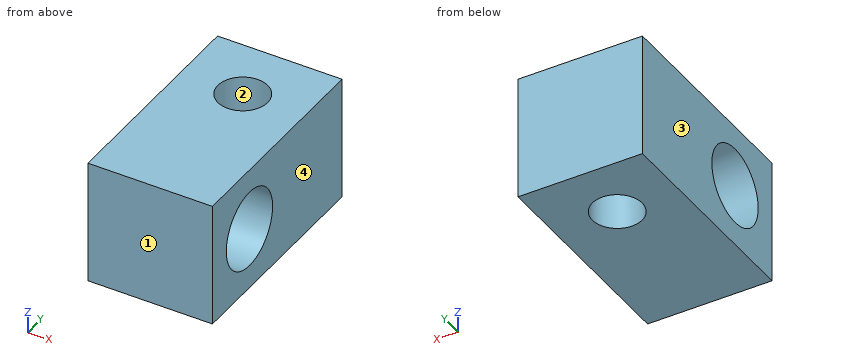
from build123d import *

# Parameters (mm, degrees)
SKETCH1_W           = 8
SKETCH1_H           = 14
BOSS_EXTRUDE1_DEPTH = 8
SKETCH2_R           = 1.6
CUT_EXTRUDE1_DEPTH  = 9
SKETCH4_R           = 2.5
CUT_EXTRUDE2_DEPTH  = 9


with BuildPart() as part:
    # Sketch1 → Boss-Extrude1 (new body)
    with BuildSketch(Plane.XY):
        Rectangle(SKETCH1_W, SKETCH1_H)
    extrude(amount=BOSS_EXTRUDE1_DEPTH)

    # Sketch2 → Cut-Extrude1 (cut, through all)
    with BuildSketch(Plane(origin=(0, 0, 0), x_dir=(-1, 0, 0), z_dir=(0, 0, -1))):
        with Locations((0, 3)):
            Circle(SKETCH2_R)
    extrude(amount=-CUT_EXTRUDE1_DEPTH, mode=Mode.SUBTRACT)

    # Sketch4 → Cut-Extrude2 (cut, through all)
    with BuildSketch(Plane.ZY.offset(4)):
        with Locations((4, -3)):
            Circle(SKETCH4_R)
    extrude(amount=-CUT_EXTRUDE2_DEPTH, mode=Mode.SUBTRACT)


solid = part.part
Read the model definition and answer for the solid it produces. Units are mm, in the model's axes. Face numbers are marked on the shaded views. Round coordinates to 2 decimals unless told otherwise and drop trailing zeros. Write each loop counter-clockwise with the first axis right and the second up, starting at its lowest first coordinate (ties: lowest second). Pieces come first, ordered by that corner, then holes. Notation, with made-up numbers: (23.5, -6.75) - (62.5, -6.75) arc R14 cw to (62.5, 11.25) - close; hole circle Ø4 at (-38, 46). An arc over 180 degrees is marked (long way). One line per question, with ' | ' between items. Start each with the question number.
1. For a pull along X with two mould halves and no side action, classify the marked faces 1, 2, 3 and 4 as +X half, -X half, draft (parallel to the pull), parting line (faces both ways), or undercut.
2. Section A-A (x = 0) is taken. Determine the outline of the cut face in (y, z).
3. Section C-C (y = -3) is taken. Determine the outline of the cut face in (x, z).
4. Find the intervals of material crossed by probe 1 along Y at (x, z) = (1.25, 4.25); probe 2 along Y at (x, z) = (0, 2.75); probe 3 along Z at (x, y) = (3.5, -4), in increasing order. Write a range as [from, to].
5. Section B-B (z = 4) is taken. Determine the outline of the cut face in (x, y), and give its area (3 significant figures).
6. Section D-D (x = 3.5) is taken. Determine the outline of the cut face in (y, z).
Filled in:
1) face 1: draft | face 2: undercut | face 3: -X half | face 4: +X half
2) outline: (-7, 0) - (1.4, 0) - (1.4, 8) - (-7, 8) - close; (4.6, 0) - (7, 0) - (7, 8) - (4.6, 8) - close; hole circle Ø5 at (-3, 4)
3) outline: (-4, 0) - (4, 0) - (4, 1.5) - (-4, 1.5) - close; (-4, 6.5) - (4, 6.5) - (4, 8) - (-4, 8) - close
4) probe 1: [-7, -5.49], [-0.51, 2], [4, 7] | probe 2: [-7, -5.17], [-0.83, 1.4], [4.6, 7] | probe 3: [0, 1.71], [6.29, 8]
5) outline: (-4, -7) - (4, -7) - (4, -5.5) - (-4, -5.5) - close; (-4, -0.5) - (4, -0.5) - (4, 7) - (-4, 7) - close; hole circle Ø3.2 at (0, 3) | area: 64.0 mm²
6) outline: (-7, 0) - (7, 0) - (7, 8) - (-7, 8) - close; hole circle Ø5 at (-3, 4)
